from build123d import *

# Parameters (mm, degrees)
CROQUIS1_R              = 1.524
SALIENTE_EXTRUIR1_DEPTH = 3.1242


with BuildPart() as part:
    # Croquis1 → Saliente-Extruir1 (new body)
    with BuildSketch(Plane.XY):
        with BuildLine():
            ThreePointArc((8.332137397, 4.338663109), (7.962691234, 4.047198075), (7.8232, 3.597771185))
            Line((7.8232, 3.597771185), (7.8232, -5.000625))
            ThreePointArc((7.8232, -5.000625), (7.706958004, -5.281258004), (7.426325, -5.3975))
            Line((7.426325, -5.3975), (-7.426325, -5.3975))
            ThreePointArc((-7.426325, -5.3975), (-7.706958004, -5.281258004), (-7.8232, -5.000625))
            Line((-7.8232, -5.000625), (-7.8232, 3.597771185))
            ThreePointArc((-7.8232, 3.597771185), (-7.962691234, 4.047198075), (-8.332137397, 4.338663109))
            ThreePointArc((-8.332137397, 4.338663109), (-12.631843868, 3.831339334), (-14.6482, 0))
            ThreePointArc((-14.6482, 0), (-15.044061243, -5.278443796), (-16.222788897, -10.4388))
            ThreePointArc((-16.222788897, -10.4388), (-16.58990766, -12.046010608), (-16.7132, -13.69))
            Line((-16.7132, -13.69), (-16.7132, -17.5))
            Line((-16.7132, -17.5), (-12.7, -17.5))
            Line((-12.7, -17.5), (-12.7, -13.69))
            Line((-12.7, -13.69), (-13.319125, -13.69))
            ThreePointArc((-13.319125, -13.69), (-13.599758004, -13.573758004), (-13.716, -13.293125))
            Line((-13.716, -13.293125), (-13.716, -12.448575))
            ThreePointArc((-13.716, -12.448575), (-13.599758004, -12.167941996), (-13.319125, -12.0517))
            Line((-13.319125, -12.0517), (-12.7, -12.0517))
            Line((-12.7, -12.0517), (-12.7, -10.835675))
            ThreePointArc((-12.7, -10.835675), (-12.583758004, -10.555041996), (-12.303125, -10.4388))
            Line((-12.303125, -10.4388), (-11.318875, -10.4388))
            ThreePointArc((-11.318875, -10.4388), (-11.038241996, -10.555041996), (-10.922, -10.835675))
            Line((-10.922, -10.835675), (-10.922, -12.0517))
            Line((-10.922, -12.0517), (-10.302875, -12.0517))
            ThreePointArc((-10.302875, -12.0517), (-10.022241996, -12.167941996), (-9.906, -12.448575))
            Line((-9.906, -12.448575), (-9.906, -13.293125))
            ThreePointArc((-9.906, -13.293125), (-10.022241996, -13.573758004), (-10.302875, -13.69))
            Line((-10.302875, -13.69), (-10.922, -13.69))
            Line((-10.922, -13.69), (-10.922, -17.5))
            Line((-10.922, -17.5), (-5.461, -17.5))
            Line((-5.461, -17.5), (-5.461, -20.6242))
            Line((-5.461, -20.6242), (5.461, -20.6242))
            Line((5.461, -20.6242), (5.461, -17.5))
            Line((5.461, -17.5), (10.922, -17.5))
            Line((10.922, -17.5), (10.922, -13.69))
            Line((10.922, -13.69), (10.302875, -13.69))
            ThreePointArc((10.302875, -13.69), (10.022241996, -13.573758004), (9.906, -13.293125))
            Line((9.906, -13.293125), (9.906, -12.448575))
            ThreePointArc((9.906, -12.448575), (10.022241996, -12.167941996), (10.302875, -12.0517))
            Line((10.302875, -12.0517), (10.922, -12.0517))
            Line((10.922, -12.0517), (10.922, -10.835675))
            ThreePointArc((10.922, -10.835675), (11.038241996, -10.555041996), (11.318875, -10.4388))
            Line((11.318875, -10.4388), (12.303125, -10.4388))
            ThreePointArc((12.303125, -10.4388), (12.583758004, -10.555041996), (12.7, -10.835675))
            Line((12.7, -10.835675), (12.7, -12.0517))
            Line((12.7, -12.0517), (13.319125, -12.0517))
            ThreePointArc((13.319125, -12.0517), (13.599758004, -12.167941996), (13.716, -12.448575))
            Line((13.716, -12.448575), (13.716, -13.293125))
            ThreePointArc((13.716, -13.293125), (13.599758004, -13.573758004), (13.319125, -13.69))
            Line((13.319125, -13.69), (12.7, -13.69))
            Line((12.7, -13.69), (12.7, -17.5))
            Line((12.7, -17.5), (16.7132, -17.5))
            Line((16.7132, -17.5), (16.7132, -13.69))
            ThreePointArc((16.7132, -13.69), (16.58990766, -12.046010608), (16.222788897, -10.4388))
            ThreePointArc((16.222788897, -10.4388), (15.044061243, -5.278443796), (14.6482, 0))
            ThreePointArc((14.6482, 0), (12.631843868, 3.831339334), (8.332137397, 4.338663109))
        make_face()
        with Locations((10, 0)):
            Circle(CROQUIS1_R, mode=Mode.SUBTRACT)
        with Locations((-10, 0)):
            Circle(CROQUIS1_R, mode=Mode.SUBTRACT)
    extrude(amount=SALIENTE_EXTRUIR1_DEPTH)


solid = part.part
Verification items for the finished model (mm, model axes). A direction names the side the tool comes from. Give positions to 0.01 mm unless a question says otherwise; leave off trailing zeros. Loops run counter-clockwise (first coordinate to the right, second up) from the corner with the lowest first, then second, coordinate; pieces in that order, holes last. Notation, with made-up numbers: (71.25, 27) - (103.25, 27) arc R20 ccw to (103.25, 47) - close; hole circle Ø10 at (53.25, -4). An arc over 180 degrees is marked (long way). Write each question's results on one line, items separated by ' | '.
1) Sectioned sample at D-D on x = 0. Record the boundary of the cut face in (y, z).
Solution:
outline: (-20.62, 0) - (-5.4, 0) - (-5.4, 3.12) - (-20.62, 3.12) - close
2) Sectioned sample at B-B on z = 2.4. Count the separate pieces of the cut face and the enclosed holes in it, plus the area to 3 significant figures.
Solution:
separate pieces: 1 | enclosed holes: 2 | area: 509 mm2
3) Depth check by flat-ended pin: P1, Ø1.6, axis at y = -1, z = 2, coming from the +X side; P2, Ø1.1, axis at x = -12, z = 2, coming from the -Y side; P3, Ø0.7, axis at y = -13, z = 1.5, coming from the +X side. Enter the tip coordinate at first touch or a pass-through.
Solution:
P1: x = 14.69 | P2: y = -10.52 | P3: x = 16.71
4) Tool access check on faces 1 (the flat face through (0, -5.398, 2)), 2 (the flat face through (12.7, -11, 2)), 3 (the flat face through (-13.716, -13, 2)), 4 (the flat face through (-5.461, -19, 2)). Record the directions out of +Z, -Z, +X, -X, +Y, -Y that give a thin tool (end or side, any length) a straight path to the whole face; none if there is none.
Solution:
face 1: +Z, -Z, +Y | face 2: +Z, -Z, -Y | face 3: +Z, -Z | face 4: +Z, -Z, -X, -Y
5) Sectioned sample at A-A on x = -9. Record the boundary of the cut face in (y, z), plus the area to 3 significant figures.
Solution:
outline: (-17.5, 0) - (-1.15, 0) - (-1.15, 3.12) - (-17.5, 3.12) - close; (1.15, 0) - (4.54, 0) - (4.54, 3.12) - (1.15, 3.12) - close | area: 61.7 mm2
6) Mould release check, pull along X, two halves, no side actions. Record for faces 5 (the flat face through (-16.713, -16, 2)), 6 (the flat face through (0, -11, 0)), 7 (the flat face through (-10.922, -16, 2)), 8 (the cylindrical face through (16.593, -12.069, 1.54)): pulls with the +X half, pulls with the -X half, needs draft (parallel to the pull), parting line crosses it, or undercut.
Solution:
face 5: pulls with the -X half | face 6: needs draft | face 7: undercut | face 8: pulls with the +X half
7) Sectioned sample at C-C on y = -18.5. Record the boundary of the cut face in (x, z).
Solution:
outline: (-5.46, 0) - (5.46, 0) - (5.46, 3.12) - (-5.46, 3.12) - close
8) Material ranges on L1, parallel to X at y = -15.5, z = 0.4; L2, parallel to Y at x = 10, z = 1.4; L3, parallel to X at y = 0.25, z = 2.6, recorded low to high. Write a range as from..to.
Solution:
L1: -16.71..-12.7, -10.92..10.92, 12.7..16.71 | L2: -17.5..-13.55, -12.19..-1.52, 1.52..4.65 | L3: -14.64..-11.5, -8.5..-7.82, 7.82..8.5, 11.5..14.64
